Can you work these out from the drawing? Everything is in mm from the part's minimum corner. A direction names the side the tool comes from. Give positions to 0.01 mm unless a question says otherwise; leave off trailing zeros. Order: outer loops, then holes, each group sorted by start corner. A loop starts at its lowest first (then second) coordinate and runs counter-clockwise, first axis right, second up. Notation, with made-up numbers: (69.5, 17.5) -> (105.5, 17.5) arc R35 ccw to (105.5, 52.5) -> close; hole circle Ø6 at (39.5, 24.5). An arc over 180 degrees is marked (long way). Answer as CSV lines item,"result". Start each with the question number.
(1) We'd pull the mould along X, two halves only. Please class the marked faces 3, 4, 5 and 6: released by +X, released by -X, zero draft, split by the parting line, or undercut.
(2) I want a section at A-A (y = 3.9). Please give me the cut outline in (x, z).
(3) Will these pins go through, and if not, where does the flat tip stop? pin 1 Ø4 at (y, z) = (1, 7.5) entering from -X; pin 2 Ø4 at (x, y) = (4.5, 3.5) entering from +Z; pin 3 Ø1.5 at (x, z) = (2, 4.5) entering from -Y; pin 4 Ø2.5 at (x, y) = (4, 4) entering from -Z.
(4) I want a section at D-D (z = 0.75). Please give me the cut outline in (x, y), plus the area to 3 significant figures.
(5) I want a section at B-B (z = 8). Please give me the cut outline in (x, y), plus the area to 3 significant figures.
(6) On a 3-axis mill with a long thin cutter (end or side, diameter ignored), from which of +Z, -Z, +X, -X, +Y, -Y can I reach the whole of each face in a straight line? I mean the marked faces 1 and 2. Say none if no direction works.
(7) I need wall thicknesses on L1, parallel to Y at x = 3.9, z = 0.5; L2, parallel to Y at x = 1.5, z = 6.5. Which ranges of each line are inside material? Lowest first, please.
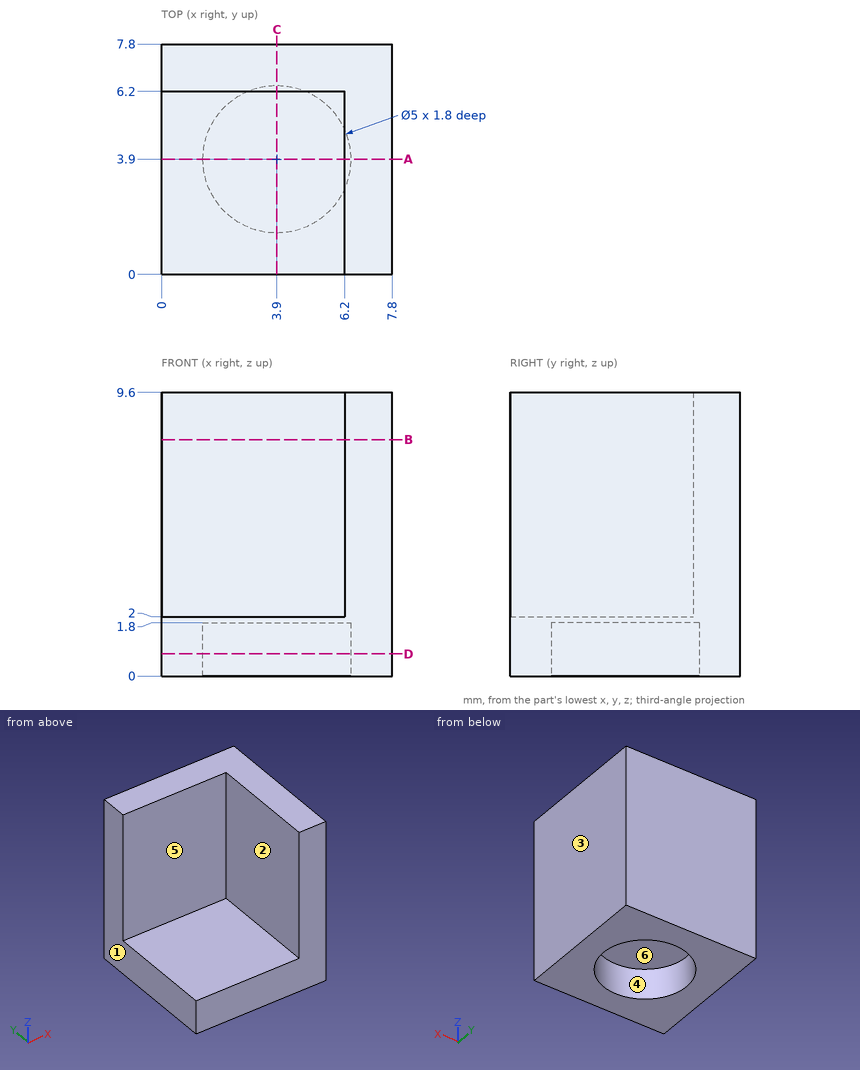
Final values:
1,face 3,"released by +X"
1,face 4,"undercut"
1,face 5,"zero draft"
1,face 6,"undercut"
2,outline,"(0, 0) -> (1.4, 0) -> (1.4, 1.8) -> (6.4, 1.8) -> (6.4, 0) -> (7.8, 0) -> (7.8, 9.6) -> (6.2, 9.6) -> (6.2, 2) -> (0, 2) -> close"
3,pin 1,"x = 6.2"
3,pin 2,"z = 9.6"
3,pin 3,"y = 6.2"
3,pin 4,"z = 1.8"
4,outline,"(0, 0) -> (7.8, 0) -> (7.8, 7.8) -> (0, 7.8) -> close; hole circle Ø5 at (3.9, 3.9)"
4,area,"41.2 mm²"
5,outline,"(0, 6.2) -> (6.2, 6.2) -> (6.2, 0) -> (7.8, 0) -> (7.8, 7.8) -> (0, 7.8) -> close"
5,area,"22.4 mm²"
6,face 1,"+Z, -Z, -X, +Y, -Y"
6,face 2,"+Z, -X, -Y"
7,L1,"0 to 1.4, 6.4 to 7.8"
7,L2,"6.2 to 7.8"
